The model under review builds one solid part; all positions refer to its coordinate system, in mm. Face numbers are marked on the shaded views. A direction names the side the tool comes from. Coordinates: 2 decimals unless noted, no trailing zeros. Write each loop counter-clockwise with the first axis right and the second up, starting at its lowest first coordinate (ties: lowest second). Pieces come first, ordered by that corner, then holes. Notation, with made-up numbers: (27.25, -13.5) - (69.25, -13.5) arc R22 cw to (69.25, -2.5) - close; hole circle Ø6 at (-4, 63.25). An arc over 180 degrees is marked (long way). Answer as CSV lines item,"result". Start each with the question number.
```python
from build123d import *

# Parameters (mm, degrees)
RESSALTO_EXTRUS_O1_DEPTH = 100
CORTE_EXTRUS_O1_DEPTH    = 51.001510114
CORTE_EXTRUS_O4_DEPTH    = 87
CORTE_EXTRUS_O6_DEPTH    = 20
CORTE_EXTRUS_O8_REACH    = 104
ESBO_O10_R               = 9
ESBO_O12_R               = 14.94
CORTE_EXTRUS_O10_DEPTH   = 24.04
CORTE_EXTRUS_O10_TAPER   = 12.85


with BuildPart() as part:
    # Esboço3 → Ressalto-extrusão1 (new body)
    with BuildSketch(Plane(origin=(0, 0, 0), x_dir=(0, 0, -1), z_dir=(1, 0, 0))):
        Polygon((0, 0), (0, -70), (-12, -80.38), (-60, -80.38), (-60, -48.378489886), (-170, -48.378489886), (-170, -30.378489886), (-115, -30.378489886), (-115, 11.621510114), (-105.001510114, 21.62), (-81.001510114, 21.62), (-69.343860018, -8.343860018), (-33.343860018, -8.343860018), (-25, 0), align=None)
    extrude(amount=RESSALTO_EXTRUS_O1_DEPTH)

    # Esboço5 → Corte-extrusão1 (cut, through all)
    with BuildSketch(Plane(origin=(0, -30.378489886, 0), x_dir=(1, 0, 0), z_dir=(0, 1, 0))):
        with BuildLine():
            Line((5, -155.02), (5, -129.98))
            ThreePointArc((5, -129.98), (12, -122.98), (19, -129.98))
            Line((19, -129.98), (19, -155.02))
            ThreePointArc((19, -155.02), (12, -162.02), (5, -155.02))
        make_face()
        with BuildLine():
            Line((29.96, -155.02), (29.96, -129.98))
            ThreePointArc((29.96, -129.98), (36.96, -122.98), (43.96, -129.98))
            Line((43.96, -129.98), (43.96, -155.02))
            ThreePointArc((43.96, -155.02), (36.96, -162.02), (29.96, -155.02))
        make_face()
        with BuildLine():
            Line((54.92, -155.02), (54.92, -129.98))
            ThreePointArc((54.92, -129.98), (61.92, -122.98), (68.92, -129.98))
            Line((68.92, -129.98), (68.92, -155.02))
            ThreePointArc((68.92, -155.02), (61.92, -162.02), (54.92, -155.02))
        make_face()
        with BuildLine():
            Line((79.88, -155.02), (79.88, -129.98))
            ThreePointArc((79.88, -129.98), (86.88, -122.98), (93.88, -129.98))
            Line((93.88, -129.98), (93.88, -155.02))
            ThreePointArc((93.88, -155.02), (86.88, -162.02), (79.88, -155.02))
        make_face()
    extrude(amount=-CORTE_EXTRUS_O1_DEPTH, mode=Mode.SUBTRACT)

    # Esboço6 → Corte-extrusão4 (cut)
    with BuildSketch(Plane(origin=(3.989809214, 22.165606742, 7.25419857), x_dir=(0.985680811, -0.160257749, -0.052447991), z_dir=(0.168621878, 0.936788213, 0.306585233))):
        Polygon((-4.047769995, -171.016408889), (97.404950637, -176.615111976), (97.404950637, -118.744566791), align=None)
    extrude(amount=CORTE_EXTRUS_O4_DEPTH, mode=Mode.SUBTRACT)

    # Esboço9 → Corte-extrusão6 (cut)
    with BuildSketch(Plane.ZY):
        Polygon((105, 11.62), (87.841109365, 11.62), (76.183459269, -18.343860018), (29.781857804, -18.343860018), (21.437997786, -10), (10, -10), (10, -65.427954016), (15.724908652, -70.38), (50, -70.38), (50, -38.378489886), (105, -38.378489886), align=None)
    extrude(amount=-CORTE_EXTRUS_O6_DEPTH, mode=Mode.SUBTRACT)

    # Esboço10 → Corte-extrusão8 (cut, up to next)
    with BuildSketch(Plane.XZ.offset(80.38), mode=Mode.PRIVATE) as corte_extrus_o8_sk1:
        with Locations((50, 50.5)):
            Circle(ESBO_O10_R)
    corte_extrus_o8_tool1 = extrude(corte_extrus_o8_sk1.sketch, amount=-CORTE_EXTRUS_O8_REACH, mode=Mode.PRIVATE) & part.part
    add(corte_extrus_o8_tool1.solids().sort_by_distance((50, -80.38, 50.5))[0], mode=Mode.SUBTRACT)

    # Esboço12 → Corte-extrusão10 (cut)
    with BuildSketch(Plane(origin=(0, -8.343860018, 0), x_dir=(1, 0, 0), z_dir=(0, 1, 0))):
        with Locations((50, -50.5)):
            Circle(ESBO_O12_R)
    extrude(amount=-CORTE_EXTRUS_O10_DEPTH, taper=CORTE_EXTRUS_O10_TAPER, mode=Mode.SUBTRACT)


solid = part.part
```
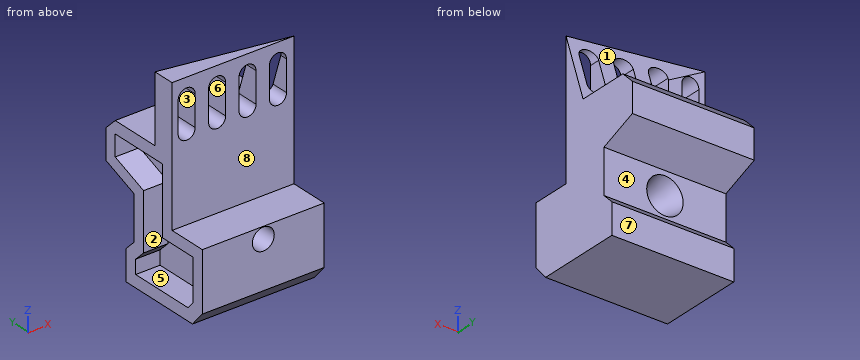
(1) Add section A-A on x = 9. Give the number of separate pieces and of enclosed holes in the cut face, then the cut area to 3 significant figures.
(2) Add section B-B on y = -56. Give the boundary of the cut face in (x, z).
(3) The part is to be moulded in two halves that separate along X. For the marked faces 1, 2 and 3, say which applies: released by +X, released by -X, zero draft, split by the parting line, or undercut.
(4) Wall thickness on line 1 (X direction, y = -30.5, z = 135.5); line 2 (Z direction, x = 50, y = -51); line 3 (Z direction, x = 43, y = -44): over which ranges is each line inside the solid? List them lowest first.
(5) For pin 1 (9.5 mm diameter, centred on x = 62, y = -56.5, fed in from +Z); pin 2 (1.5 mm diameter, centred on y = -43.5, z = 144.5, fed in from -X); pin 3 (8 mm diameter, centred on x = 78.5, z = 127.5, fed in from +Y); pin 4 (12.5 mm diameter, centred on x = 45.5, y = -15, fed in from +Z), all flat-tipped, find the tip position at first contact; note any pin that passes through.
(6) Add section D-D on x = 75.5. Give the boundary of the cut face in (y, z) (3 decimals).
(7) Add section C-C on x = 50. Give the boundary of the cut face in (y, z), then the cut area to 3 significant figures.
(8) For the marked faces 4, 5, 6, 7 and 8, list the 3-axis set-ups (+Z, -Z, +X, -X, +Y, -Y) from which the entire face can be reached by the end or side of a thin tool; tool diameter is ignored.
Reported:
1,separate pieces,"2"
1,enclosed holes,"1"
1,area,"4,170 mm²"
2,outline,"(0, 0) - (100, 0) - (100, 60) - (0, 60) - (0, 50) - (20, 50) - (20, 10) - (0, 10) - close; hole circle Ø18 at (50, 50.5)"
3,face 1,"released by +X"
3,face 2,"zero draft"
3,face 3,"undercut"
4,line 1,"0 to 5, 19 to 29.96, 43.96 to 54.92"
4,line 2,"0 to 41.5, 59.5 to 60"
4,line 3,"0 to 44.84, 56.16 to 126.44, 158.56 to 170"
5,pin 1,"z = 60"
5,pin 2,"x = 0"
5,pin 3,"y = -30.38"
5,pin 4,"z = 115"
6,outline,"(-80.38, 12) - (-70, 0) - (0, 0) - (0, 25) - (-8.344, 33.344) - (-8.344, 69.344) - (21.62, 81.002) - (21.62, 105.002) - (11.622, 115) - (-30.378, 115) - (-30.378, 128.475) - (-43.968, 170) - (-48.378, 170) - (-48.378, 60) - (-80.38, 60) - close"
7,outline,"(-80.38, 12) - (-70, 0) - (0, 0) - (0, 25) - (-8.34, 33.34) - (-8.34, 35.56) - (-32.38, 41.04) - (-32.38, 41.5) - (-80.38, 41.5) - close; (-80.38, 59.5) - (-32.38, 59.5) - (-32.38, 59.96) - (-8.34, 65.44) - (-8.34, 69.34) - (21.62, 81) - (21.62, 105) - (11.62, 115) - (-30.38, 115) - (-30.38, 142.5) - (-39.38, 170) - (-48.38, 170) - (-48.38, 60) - (-80.38, 60) - close"
7,area,"7,260 mm²"
8,face 4,"+X, -X, +Y"
8,face 5,"-X"
8,face 6,"+Y, -Y"
8,face 7,"-Z, +X, -X, +Y"
8,face 8,"+Z, +X, -X, -Y"
